Source: CAD feature listing. Evaluate the final solid. Frame: model axes, mm. Face numbers are marked on the shaded views. A direction names the side the tool comes from. Round coordinates to 2 decimals unless told otherwise and drop trailing zeros. Loops run counter-clockwise (first coordinate to the right, second up) from the corner with the lowest first, then second, coordinate; pieces in that order, holes last.
(1) Section B-B, the plane y = 38. Return the cut outline in (x, z).
(2) Section D-D, the plane y = 101. Return the cut outline in (x, z), plus the area to 3 significant figures.
(3) First-contact query: pin 1 Ø1 at (y, z) = (55, -4) entering from +X; pin 2 Ø3.5 at (y, z) = (4, -0.5) entering from -X; pin 3 Ø1.5 at (y, z) = (58, -3.5) entering from -X. Flat tips, straight axial feed; report the tip coordinate or a pass-through.
(4) Section C-C, the plane y = 134. Count the separate pieces of the cut face and the enclosed holes in it, plus the area to 3 significant figures.
(5) Section A-A, the plane z = 0.75. Return the cut outline in (x, y).
(6) Set-up query: the marked faces 1 and 2. Return all of +Z, -Z, +X, -X, +Y, -Y with unobstructed straight access to the full face (end or side cutting, diameter ignored); none if empty.
(7) Material intervals for probe 1 along X at (y, z) = (121, -4); probe 2 along X at (y, z) = (138, 0.75); probe 3 along Z at (x, y) = (-27.5, 136), sorted ascending.
(8) Mould query, pull axis X, two halves, no side actions, for the marked faces 3, 4 and 5. Classes: pulls with the +X half, pulls with the -X half, needs draft (parallel to the pull), parting line crosses it, or undercut.
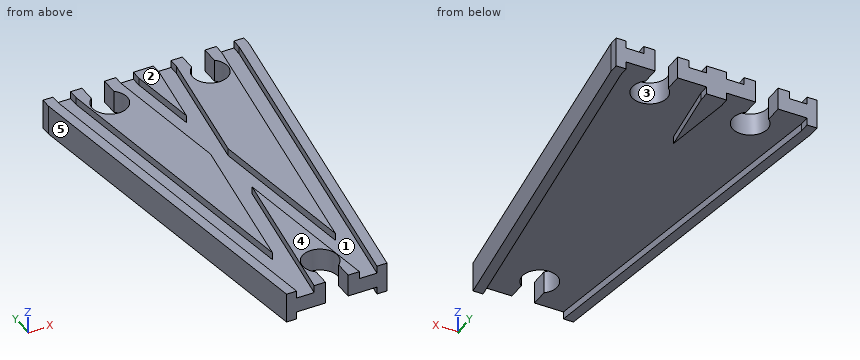
```python
from build123d import *

# Parameters (mm, degrees)
SKETCH004_W          = 32
SKETCH004_H          = 3
SKETCH005_W          = 7
SKETCH005_H          = 3
SKETCH006_W          = 7
SKETCH006_H          = 3
POCKET_DEPTH         = 6.001
POCKET_DEPTH_BACK    = -6.001
POCKET001_DEPTH      = 6.001
POCKET001_DEPTH_BACK = -6.001
POCKET002_DEPTH      = 6.001
POCKET002_DEPTH_BACK = -6.001


with BuildPart() as part:
    # AdditivePipe: sweep along a path in Sketch
    with BuildLine(Plane.XY) as additivepipe_path:
        Line((-20, 144), (-20, 140))
        Line((-20, 140), (0, 0))
    # Sketch002 → AdditivePipe (sweep)
    with BuildSketch(Plane.XZ):
        Polygon((-20, 6), (-20, -6), (-16, -6), (-16, -3), (-9, -3), (9, -3), (16, -3), (16, -6), (20, -6), (20, 6), (16, 6), (16, 3), (9, 3), (9, 6), (-9, 6), (-9, 3), (-16, 3), (-16, 6), align=None)
    sweep(path=additivepipe_path.line)

    # AdditivePipe001: sweep along a path in Sketch001
    with BuildLine(Plane.XY) as additivepipe001_path:
        Line((20, 144), (20, 140))
        Line((20, 140), (0, 0))
    # Sketch002 → AdditivePipe001 (sweep)
    with BuildSketch(Plane.XZ):
        Polygon((-20, 6), (-20, -6), (-16, -6), (-16, -3), (-9, -3), (9, -3), (16, -3), (16, -6), (20, -6), (20, 6), (16, 6), (16, 3), (9, 3), (9, 6), (-9, 6), (-9, 3), (-16, 3), (-16, 6), align=None)
    sweep(path=additivepipe001_path.line)

    # SubtractivePipe: sweep along a path in Sketch
    with BuildLine(Plane.XY) as subtractivepipe_path:
        Line((-20, 144), (-20, 140))
        Line((-20, 140), (0, 0))
    # Sketch004 → SubtractivePipe (sweep, cut)
    with BuildSketch(Plane.XZ):
        with Locations((0, -4.5)):
            Rectangle(SKETCH004_W, SKETCH004_H)
    sweep(path=subtractivepipe_path.line, mode=Mode.SUBTRACT)

    # SubtractivePipe001: sweep along a path in Sketch001
    with BuildLine(Plane.XY) as subtractivepipe001_path:
        Line((20, 144), (20, 140))
        Line((20, 140), (0, 0))
    # Sketch004 → SubtractivePipe001 (sweep, cut)
    with BuildSketch(Plane.XZ):
        with Locations((0, -4.5)):
            Rectangle(SKETCH004_W, SKETCH004_H)
    sweep(path=subtractivepipe001_path.line, mode=Mode.SUBTRACT)

    # SubtractivePipe002: sweep along a path in Sketch
    with BuildLine(Plane.XY) as subtractivepipe002_path:
        Line((-20, 144), (-20, 140))
        Line((-20, 140), (0, 0))
    # Sketch005 → SubtractivePipe002 (sweep, cut)
    with BuildSketch(Plane.XZ):
        with Locations((-12.5, 4.5)):
            Rectangle(SKETCH005_W, SKETCH005_H)
    sweep(path=subtractivepipe002_path.line, mode=Mode.SUBTRACT)

    # SubtractivePipe003: sweep along a path in Sketch001
    with BuildLine(Plane.XY) as subtractivepipe003_path:
        Line((20, 144), (20, 140))
        Line((20, 140), (0, 0))
    # Sketch005 → SubtractivePipe003 (sweep, cut)
    with BuildSketch(Plane.XZ):
        with Locations((-12.5, 4.5)):
            Rectangle(SKETCH005_W, SKETCH005_H)
    sweep(path=subtractivepipe003_path.line, mode=Mode.SUBTRACT)

    # SubtractivePipe004: sweep along a path in Sketch
    with BuildLine(Plane.XY) as subtractivepipe004_path:
        Line((-20, 144), (-20, 140))
        Line((-20, 140), (0, 0))
    # Sketch006 → SubtractivePipe004 (sweep, cut)
    with BuildSketch(Plane.XZ):
        with Locations((12.5, 4.5)):
            Rectangle(SKETCH006_W, SKETCH006_H)
    sweep(path=subtractivepipe004_path.line, mode=Mode.SUBTRACT)

    # SubtractivePipe005: sweep along a path in Sketch001
    with BuildLine(Plane.XY) as subtractivepipe005_path:
        Line((20, 144), (20, 140))
        Line((20, 140), (0, 0))
    # Sketch006 → SubtractivePipe005 (sweep, cut)
    with BuildSketch(Plane.XZ):
        with Locations((12.5, 4.5)):
            Rectangle(SKETCH006_W, SKETCH006_H)
    sweep(path=subtractivepipe005_path.line, mode=Mode.SUBTRACT)

    # Sketch003 → Pocket (cut, two sides)
    with BuildSketch(Plane.XY) as pocket_sk:
        with BuildLine():
            Line((-4.5, 0), (4.5, 0))
            Line((4.5, 0), (4.5, 7))
            ThreePointArc((4.5, 7), (0, 19.361903), (-4.5, 7))
            Line((-4.5, 0), (-4.5, 7))
        make_face()
    extrude(amount=-POCKET_DEPTH, mode=Mode.SUBTRACT)
    extrude(pocket_sk.sketch, amount=-POCKET_DEPTH_BACK, mode=Mode.SUBTRACT)

    # Sketch007 → Pocket001 (cut, two sides)
    with BuildSketch(Plane.XY) as pocket001_sk:
        with BuildLine():
            Line((-24.5, 144), (-15.5, 144))
            Line((-15.5, 144), (-15.5, 137))
            ThreePointArc((-24.5, 137), (-20, 124.638097), (-15.5, 137))
            Line((-24.5, 144), (-24.5, 137))
        make_face()
    extrude(amount=-POCKET001_DEPTH, mode=Mode.SUBTRACT)
    extrude(pocket001_sk.sketch, amount=-POCKET001_DEPTH_BACK, mode=Mode.SUBTRACT)

    # Sketch008 → Pocket002 (cut, two sides)
    with BuildSketch(Plane.XY) as pocket002_sk:
        with BuildLine():
            Line((15.5, 144), (24.5, 144))
            Line((24.5, 144), (24.5, 137))
            ThreePointArc((15.5, 137), (20, 124.638097), (24.5, 137))
            Line((15.5, 144), (15.5, 137))
        make_face()
    extrude(amount=-POCKET002_DEPTH, mode=Mode.SUBTRACT)
    extrude(pocket002_sk.sketch, amount=-POCKET002_DEPTH_BACK, mode=Mode.SUBTRACT)


solid = part.part
```
Output values:
1. outline: (-25.43, -6) - (-21.43, -6) - (-21.43, -3) - (21.43, -3) - (21.43, -6) - (25.43, -6) - (25.43, 6) - (21.43, 6) - (21.43, 3) - (14.43, 3) - (14.43, 6) - (10.57, 6) - (10.57, 3) - (3.57, 3) - (3.57, 6) - (-3.57, 6) - (-3.57, 3) - (-10.57, 3) - (-10.57, 6) - (-14.43, 6) - (-14.43, 3) - (-21.43, 3) - (-21.43, 6) - (-25.43, 6) - close
2. outline: (-34.43, -6) - (-30.43, -6) - (-30.43, -3) - (30.43, -3) - (30.43, -6) - (34.43, -6) - (34.43, 6) - (30.43, 6) - (30.43, 3) - (23.43, 3) - (23.43, 6) - (5.43, 6) - (5.43, 3) - (-5.43, 3) - (-5.43, 6) - (-23.43, 6) - (-23.43, 3) - (-30.43, 3) - (-30.43, 6) - (-34.43, 6) - close
2. area: 569 mm2
3. pin 1: stops at x = 27.93
3. pin 2: stops at x = -20.82
3. pin 3: stops at x = -28.39
4. separate pieces: 3
4. enclosed holes: 0
4. area: 426 mm2
5. outline: (-40, 140) - (-20, 0) - (-4.5, 0) - (-4.5, 7) arc R7 cw (long way) to (4.5, 7) - (4.5, 0) - (20, 0) - (40, 140) - (40, 144) - (24.5, 144) - (24.5, 137) arc R7 cw (long way) to (15.5, 137) - (15.5, 144) - (-15.5, 144) - (-15.5, 137) arc R7 cw (long way) to (-24.5, 137) - (-24.5, 144) - (-40, 144) - close
6. face 1: +Z
6. face 2: +Z, +X, -X, +Y, -Y
7. probe 1: x = -37.29 to -33.29, -1.29 to 1.29, 33.29 to 37.29
7. probe 2: x = -39.71 to -24.5, -15.5 to 15.5, 24.5 to 39.71
7. probe 3: z = -3 to 6
8. face 3: undercut
8. face 4: needs draft
8. face 5: pulls with the -X half
